from build123d import *

# Parameters (mm, degrees)
PAD026_DEPTH            = 1.5
SKETCH032_R             = 1
POCKET005_DEPTH         = 1.501
PAD027_DEPTH            = 13.5
FILLET001_R             = 2
CHAMFER004_SIZE2        = 11
CHAMFER004_SIZE         = 5.5
SKETCH034_R             = 7.5
PAD028_DEPTH            = 10.5
SKETCH035_R             = 2.5
PAD029_DEPTH            = 1
SKETCH036_W             = 2
SKETCH036_H             = 13.5
PAD030_DEPTH            = 60
SKETCH037_R             = 1.75
PAD031_DEPTH            = 4
SKETCH038_R             = 4
PAD032_DEPTH            = 50
SKETCH039_R             = 1.75
PAD033_DEPTH            = 6
BODY011_ROLL_ANGLE      = 180
BODY011_PLACEMENT_ANGLE = 90


with BuildPart() as part:
    # Sketch031 → Pad026 (new body)
    with BuildSketch(Plane.XY):
        with BuildLine():
            Line((0, 0), (69, 0))
            Line((69, 0), (69, 19))
            ThreePointArc((69, 19), (68.414214, 20.414214), (67, 21))
            Line((67, 21), (9, 21))
            Line((9, 21), (9, 33))
            Line((9, 33), (4, 33))
            ThreePointArc((4, 33), (2.585786, 32.414214), (2, 31))
            Line((2, 31), (2, 24.5))
            Line((2, 24.5), (1, 24.5))
            Line((1, 24.5), (0, 22))
            Line((0, 0), (0, 22))
        make_face()
    extrude(amount=PAD026_DEPTH)

    # Sketch032 (on Face13 of Pad026) → Pocket005 (cut, through all)
    with BuildSketch(Plane.XY.offset(1.5)):
        with Locations((4, 31)):
            Circle(SKETCH032_R)
        with BuildLine():
            ThreePointArc((67, 18), (68, 19), (67, 20))
            Line((67, 20), (66.5, 20))
            ThreePointArc((66.5, 20), (65.5, 19), (66.5, 18))
            Line((67, 18), (66.5, 18))
        make_face()
    extrude(amount=-POCKET005_DEPTH, mode=Mode.SUBTRACT)

    # Sketch033 (on Face4 of Pocket005) → Pad027 (join)
    with BuildSketch(Plane(origin=(0, 0, 0), x_dir=(1, 0, 0), z_dir=(0, 0, -1))):
        Polygon((69, -16.5), (9, -16.5), (9, -33), (7, -33), (7, -28), (2, -28), (0, -22), (0, 0), (9, 0), (9, -13.5), (67.5, -13.5), (67.5, 0), (69, 0), align=None)
    extrude(amount=PAD027_DEPTH)

    # Fillet001
    fillet001_edges = [part.edges().sort_by_distance(p)[0] for p in [
        (4.5, 28, -13.5),
    ]]
    fillet(fillet001_edges, radius=FILLET001_R)

    # Chamfer004
    chamfer004_edges = [part.edges().sort_by_distance(p)[0] for p in [
        (8, 33, -13.5),
    ]]
    chamfer004_side = part.faces().sort_by_distance((21.468212, 13.972492, -13.5))[0]
    chamfer(chamfer004_edges, length=CHAMFER004_SIZE, length2=CHAMFER004_SIZE2, reference=chamfer004_side)

    # Sketch034 (on Face5 of Chamfer004) → Pad028 (join)
    with BuildSketch(Plane.YZ.offset(9)):
        with Locations((25.5, -6)):
            Circle(SKETCH034_R)
    extrude(amount=PAD028_DEPTH)

    # Sketch035 (on Face1 of Pad028) → Pad029 (join)
    with BuildSketch(Plane.YZ.offset(19.5)):
        with Locations((25.5, -6)):
            Circle(SKETCH035_R)
    extrude(amount=PAD029_DEPTH)

    # Sketch036 (on Face23 of Pad029) → Pad030 (join)
    with BuildSketch(Plane.YZ.offset(9)):
        with Locations((10.5, -6.75)):
            Rectangle(SKETCH036_W, SKETCH036_H)
    extrude(amount=PAD030_DEPTH)

    # Sketch037 (on Face1 of Pad030) → Pad031 (join)
    with BuildSketch(Plane.YZ.offset(9)):
        with Locations((6, -9)):
            Circle(SKETCH037_R)
    extrude(amount=PAD031_DEPTH)

    # Sketch038 (on Face22 of Pad031) → Pad032 (join)
    with BuildSketch(Plane.YZ.offset(13)):
        with Locations((6, -9)):
            Circle(SKETCH038_R)
    extrude(amount=PAD032_DEPTH)

    # Sketch039 (on Face8 of Pad032) → Pad033 (join)
    with BuildSketch(Plane.YZ.offset(63)):
        with Locations((6, -9)):
            Circle(SKETCH039_R)
    extrude(amount=PAD033_DEPTH)


with BuildPart() as part_1:
    # Body011 roll: moved
    add(part.part.rotate(Axis((0, 0, 0), (1, 0, 0)), BODY011_ROLL_ANGLE))


with BuildPart() as part_2:
    # Body011 placement: moved
    add(part_1.part.moved(Location((-196, 277, 54.5))).rotate(Axis((-196, 277, 54.5), (0, 0, 1)), BODY011_PLACEMENT_ANGLE))


solid = part_2.part
Geometry check sheet. Reference: the model listing, model coordinates, mm. A direction names the side the tool comes from. Round coordinates to 2 decimals unless told otherwise and drop trailing zeros. Write each loop counter-clockwise with the first axis right and the second up, starting at its lowest first coordinate (ties: lowest second). Pieces come first, ordered by that corner, then holes.
Item 1: Access from +Z, -Z, +X, -X, +Y, -Y to the whole of each face (thin tool, end or side, straight path). Record for faces 4 (the face through (-191, 315, 54.5)), 5 (the face through (-188.331, 342.218, 62.974)), 6 (the face through (-165.7, 285, 62.4)).
Determined:
face 4: -X
face 5: none
face 6: +Z, +X, -Y
Item 2: Section check A-A (x = -190). Record the boundary of the cut face in (y, z).
Determined:
outline: (277, 53) - (346, 53) - (346, 68) - (344.5, 68) - (344.5, 65.25) - (340, 65.25) - (340, 67.5) - (290, 67.5) - (290, 65.25) - (286, 65.25) - (286, 68) - (277, 68) - close; hole (286, 54.5) - (344.5, 54.5) - (344.5, 61.75) - (340, 61.75) - (340, 59.5) - (290, 59.5) - (290, 61.75) - (286, 61.75) - close
Item 3: Go/stop test with flat-tipped pins: pin 1 Ø2.5 at (x, z) = (-165.5, 54.5) entering from +Y; pin 2 Ø2.5 at (x, z) = (-166, 61) entering from -Y; pin 3 Ø0.6 at (x, y) = (-183.5, 307.5) entering from +Z. Record where each tip stops, or that it passes through.
Determined:
pin 1: stops at y = 296.5
pin 2: stops at y = 284
pin 3: stops at z = 54.5
Item 4: Mould release check, pull along Z, two halves, no side actions. Record for faces 1 (the face through (-191, 344.5, 61)), 2 (the face through (-168.115, 296.993, 59.749)), 3 (the face through (-183, 315, 54.5)): +Z half, -Z half, draft (parallel to the pull), parting line (faces both ways), or undercut.
Determined:
face 1: undercut
face 2: parting line
face 3: +Z half
Item 5: Material ranges on line 1 along Y through (x, z) = (-165, 53.4); line 2 along X through (y, z) = (343, 56.25); line 3 along X through (y, z) = (281, 53.4), recorded low to high.
Determined:
line 1: y = 279 to 280, 282 to 286
line 2: x = -186.5 to -184.5, -182.5 to -179.5
line 3: x = -196 to -166, -164 to -163
Item 6: Section check B-B (y = 306.5). Record the boundary of the cut face in (x, z), plus the area to 3 significant figures.
Determined:
outline: (-196, 53) - (-175, 53) - (-175, 54.5) - (-179.5, 54.5) - (-179.5, 68) - (-182.5, 68) - (-182.5, 54.5) - (-184.5, 54.5) - (-184.5, 68) - (-186.5, 68) - (-186.5, 65.44) arc R4 ccw (long way) to (-186.5, 61.56) - (-186.5, 54.5) - (-196, 54.5) - close
area: 148 mm2
